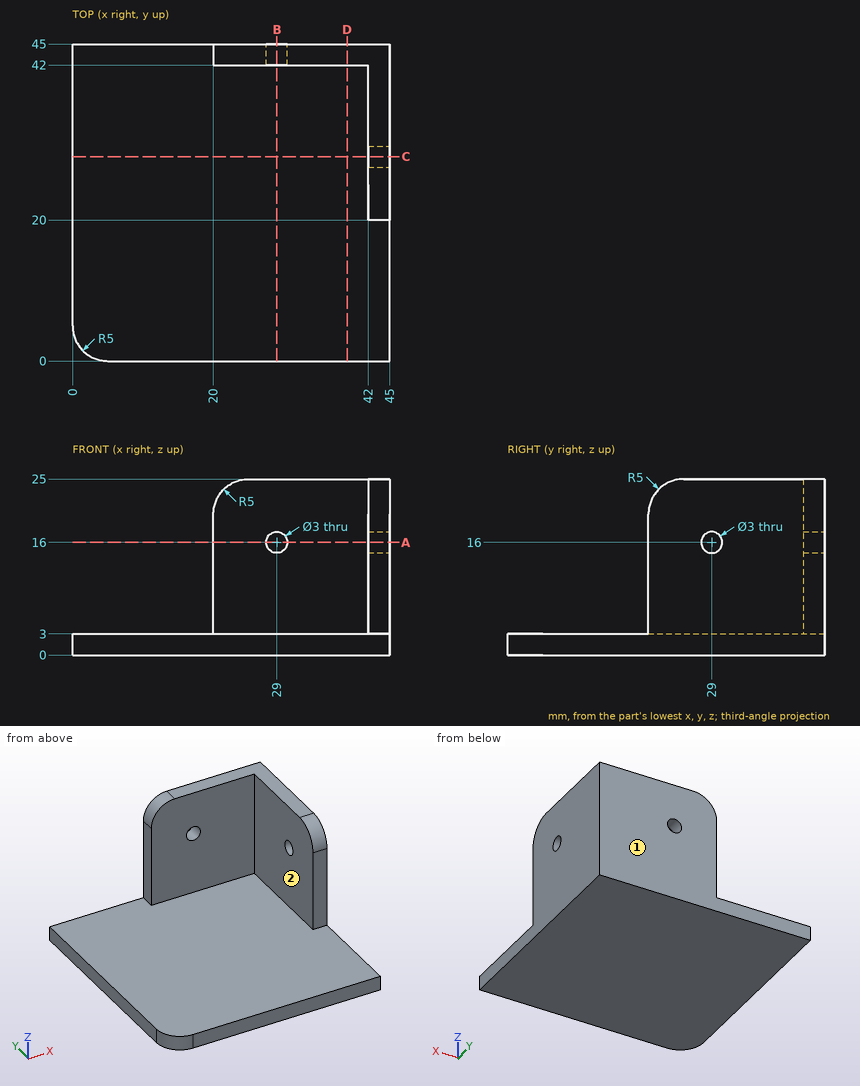
Input: dimensioned drawing with shaded views. Units: mm. Origin: part minimum x, y, z. A direction names the side the tool comes from. Coordinates: 2 decimals unless noted, no trailing zeros. Loops run counter-clockwise (first coordinate to the right, second up) from the corner with the lowest first, then second, coordinate; pieces in that order, holes last. Notation, with made-up numbers: M 88.25,-0.75 L 130.25,-0.75 A32 cw 130.25,33.25 Z; hole C -15,58.25 d5. An arc over 180 degrees is marked long. One line per item, written item: value. Start each with the question number.
1) Pin query (flat end, axial travel): P1, Ø2.5, axis at y = 29, z = 16, coming from the -X side; P2, Ø12, axis at x = 35, z = 20, coming from the -Y side; P3, Ø2.5, axis at y = 44, z = 7.5, coming from the -X side; P4, Ø10, axis at x = 13.5, y = 5, coming from the +Z side. Return the tip coordinate at first contact, or that it passes through.
2) Reachability of the marked faces 1 and 2 from +Z, -Z, +X, -X, +Y, -Y: full face, straight path, thin tool, end or side. Return the list, or none.
3) Cut plane D-D (x = 39). Return loops of the section in (y, z).
4) Cut plane A-A (z = 16). Return loops of the section in (x, y).
5) Cut plane B-B (x = 29). Return loops of the section in (y, z), then the cut area to 3 significant figures.
6) Material intervals for L1, parallel to Z at x = 44, y = 29; L2, parallel to Z at x = 21, y = 10.5; L3, parallel to X at y = 23.5, z = 8.5, sorted ascending. Write a range as from..to.
Evaluation:
1. P1: through
1. P2: y = 42
1. P3: x = 20
1. P4: z = 3
2. face 1: +Z, -Z, +X, -X, +Y
2. face 2: +Z, -X, -Y
3. outline: M 0,0 L 45,0 L 45,25 L 42,25 L 42,3 L 0,3 Z
4. outline: M 20,42 L 27.5,42 L 27.5,45 L 20,45 Z; M 30.5,42 L 42,42 L 42,30.5 L 45,30.5 L 45,45 L 30.5,45 Z; M 42,20 L 45,20 L 45,27.5 L 42,27.5 Z
5. outline: M 0,0 L 45,0 L 45,14.5 L 42,14.5 L 42,3 L 0,3 Z; M 42,17.5 L 45,17.5 L 45,25 L 42,25 Z
5. area: 192 mm^2
6. L1: 0..14.5, 17.5..25
6. L2: 0..3
6. L3: 42..45
